```python
from build123d import *

# Parameters (mm, degrees)
F0_R     = 1.5
F1_DEPTH = 2.8448
F2_DEPTH = 1.3208
F3_DEPTH = 0.381
F4_DEPTH = 2.8458


with BuildPart() as f1:
    # F0 (on Top) → F1 (new body)
    with BuildSketch(Plane.XY):
        with BuildLine():
            Line((11.4554, 2.2225), (-11.4554, 2.2225))
            ThreePointArc((-11.4554, 2.2225), (-12.896206, 1.39065), (-12.896206, -0.27305))
            Line((-12.896206, -0.27305), (-12.25096, -1.39065))
            ThreePointArc((-12.25096, -1.39065), (-11.642003, -1.999606), (-10.810153, -2.2225))
            Line((-10.810153, -2.2225), (10.810153, -2.2225))
            ThreePointArc((10.810153, -2.2225), (11.642003, -1.999606), (12.25096, -1.39065))
            Line((12.25096, -1.39065), (12.896206, -0.27305))
            ThreePointArc((12.896206, -0.27305), (12.896206, 1.39065), (11.4554, 2.2225))
        make_face()
        with BuildLine():
            ThreePointArc((-12.566251, -0.08255), (-12.566251, 1.20015), (-11.4554, 1.8415))
            Line((-11.4554, 1.8415), (11.4554, 1.8415))
            ThreePointArc((11.4554, 1.8415), (12.566251, 1.20015), (12.566251, -0.08255))
            Line((12.566251, -0.08255), (11.921004, -1.20015))
            ThreePointArc((11.921004, -1.20015), (11.451503, -1.669651), (10.810153, -1.8415))
            Line((10.810153, -1.8415), (-10.810153, -1.8415))
            ThreePointArc((-10.810153, -1.8415), (-11.451503, -1.669651), (-11.921004, -1.20015))
            Line((-11.921004, -1.20015), (-12.566251, -0.08255))
        make_face(mode=Mode.SUBTRACT)
        with BuildLine():
            Line((11.4554, 1.8415), (-11.4554, 1.8415))
            ThreePointArc((-11.4554, 1.8415), (-12.566251, 1.20015), (-12.566251, -0.08255))
            Line((-12.566251, -0.08255), (-11.921004, -1.20015))
            ThreePointArc((-11.921004, -1.20015), (-11.451503, -1.669651), (-10.810153, -1.8415))
            Line((-10.810153, -1.8415), (10.810153, -1.8415))
            ThreePointArc((10.810153, -1.8415), (11.451503, -1.669651), (11.921004, -1.20015))
            Line((11.921004, -1.20015), (12.566251, -0.08255))
            ThreePointArc((12.566251, -0.08255), (12.566251, 1.20015), (11.4554, 1.8415))
        make_face()
        with BuildLine():
            ThreePointArc((-12.34628, 0.04445), (-12.34628, 1.07315), (-11.4554, 1.5875))
            Line((-11.4554, 1.5875), (11.4554, 1.5875))
            ThreePointArc((11.4554, 1.5875), (12.34628, 1.07315), (12.34628, 0.04445))
            Line((12.34628, 0.04445), (11.701034, -1.07315))
            ThreePointArc((11.701034, -1.07315), (11.324503, -1.44968), (10.810153, -1.5875))
            Line((10.810153, -1.5875), (-10.810153, -1.5875))
            ThreePointArc((-10.810153, -1.5875), (-11.324503, -1.44968), (-11.701034, -1.07315))
            Line((-11.701034, -1.07315), (-12.34628, 0.04445))
        make_face(mode=Mode.SUBTRACT)
        with BuildLine():
            Line((11.4554, 1.5875), (-11.4554, 1.5875))
            ThreePointArc((-11.4554, 1.5875), (-12.34628, 1.07315), (-12.34628, 0.04445))
            Line((-12.34628, 0.04445), (-11.701034, -1.07315))
            ThreePointArc((-11.701034, -1.07315), (-11.324503, -1.44968), (-10.810153, -1.5875))
            Line((-10.810153, -1.5875), (10.810153, -1.5875))
            ThreePointArc((10.810153, -1.5875), (11.324503, -1.44968), (11.701034, -1.07315))
            Line((11.701034, -1.07315), (12.34628, 0.04445))
            ThreePointArc((12.34628, 0.04445), (12.34628, 1.07315), (11.4554, 1.5875))
        make_face()
        with Locations((-10.500578, 0)):
            Circle(F0_R, mode=Mode.SUBTRACT)
        with Locations((10.500578, 0)):
            Circle(F0_R, mode=Mode.SUBTRACT)
        with Locations((-10.500578, 0)):
            Circle(F0_R)
        with Locations((10.500578, 0)):
            Circle(F0_R)
    extrude(amount=-F1_DEPTH)

    # F0 (on Top) → F2 (cut)
    with BuildSketch(Plane.XY):
        with BuildLine():
            Line((11.4554, 1.5875), (-11.4554, 1.5875))
            ThreePointArc((-11.4554, 1.5875), (-12.34628, 1.07315), (-12.34628, 0.04445))
            Line((-12.34628, 0.04445), (-11.701034, -1.07315))
            ThreePointArc((-11.701034, -1.07315), (-11.324503, -1.44968), (-10.810153, -1.5875))
            Line((-10.810153, -1.5875), (10.810153, -1.5875))
            ThreePointArc((10.810153, -1.5875), (11.324503, -1.44968), (11.701034, -1.07315))
            Line((11.701034, -1.07315), (12.34628, 0.04445))
            ThreePointArc((12.34628, 0.04445), (12.34628, 1.07315), (11.4554, 1.5875))
        make_face()
        with Locations((-10.500578, 0)):
            Circle(F0_R, mode=Mode.SUBTRACT)
        with Locations((10.500578, 0)):
            Circle(F0_R, mode=Mode.SUBTRACT)
        with Locations((-10.500578, 0)):
            Circle(F0_R)
        with Locations((10.500578, 0)):
            Circle(F0_R)
    extrude(amount=-F2_DEPTH, mode=Mode.SUBTRACT)

    # F0 (on Top) → F3 (cut)
    with BuildSketch(Plane.XY):
        with BuildLine():
            Line((11.4554, 1.8415), (-11.4554, 1.8415))
            ThreePointArc((-11.4554, 1.8415), (-12.566251, 1.20015), (-12.566251, -0.08255))
            Line((-12.566251, -0.08255), (-11.921004, -1.20015))
            ThreePointArc((-11.921004, -1.20015), (-11.451503, -1.669651), (-10.810153, -1.8415))
            Line((-10.810153, -1.8415), (10.810153, -1.8415))
            ThreePointArc((10.810153, -1.8415), (11.451503, -1.669651), (11.921004, -1.20015))
            Line((11.921004, -1.20015), (12.566251, -0.08255))
            ThreePointArc((12.566251, -0.08255), (12.566251, 1.20015), (11.4554, 1.8415))
        make_face()
        with BuildLine():
            ThreePointArc((-12.34628, 0.04445), (-12.34628, 1.07315), (-11.4554, 1.5875))
            Line((-11.4554, 1.5875), (11.4554, 1.5875))
            ThreePointArc((11.4554, 1.5875), (12.34628, 1.07315), (12.34628, 0.04445))
            Line((12.34628, 0.04445), (11.701034, -1.07315))
            ThreePointArc((11.701034, -1.07315), (11.324503, -1.44968), (10.810153, -1.5875))
            Line((10.810153, -1.5875), (-10.810153, -1.5875))
            ThreePointArc((-10.810153, -1.5875), (-11.324503, -1.44968), (-11.701034, -1.07315))
            Line((-11.701034, -1.07315), (-12.34628, 0.04445))
        make_face(mode=Mode.SUBTRACT)
    extrude(amount=-F3_DEPTH, mode=Mode.SUBTRACT)

    # F0 (on Top) → F4 (cut, through all)
    with BuildSketch(Plane.XY):
        with Locations((-10.500578, 0)):
            Circle(F0_R)
        with Locations((10.500578, 0)):
            Circle(F0_R)
    extrude(amount=-F4_DEPTH, mode=Mode.SUBTRACT)


solid = f1.part
```
Work out the finished part from the listing and answer in its coordinate system (mm). A direction names the side the tool comes from. Round coordinates to 2 decimals unless told otherwise and drop trailing zeros. Write each loop counter-clockwise with the first axis right and the second up, starting at its lowest first coordinate (ties: lowest second). Pieces come first, ordered by that corner, then holes. Notation, with made-up numbers: (-22.5, 7) - (21.5, 7) arc R11 cw to (21.5, 22) - close; hole circle Ø4 at (47, -30.5). An arc over 180 degrees is marked (long way). Return JSON: item names as keys, results as strings. Group by question number.
Q1. Find the intervals of material crossed by L1, parallel to Y at x = 10.5, z = -1.45; L2, parallel to X at y = 1.2, z = -2.35; L3, parallel to Y at x = 8, z = -1, in increasing order.
Q2. The part is cut by section A-A on z = -2.3. Write down the section's boundary in (x, y), then the cut area to 3 significant figures.
Q3. The part is cut by section C-C on y = 1.15. Write down the section's boundary in (x, z).
Q4. The part is cut by section B-B on x = -8.5. Write down the section's boundary in (y, z).
Q5. The part is cut by section D-D on y = -0.55. Write down the section's boundary in (x, z), then the cut area to 3 significant figures.
Q6. Each of these flat-tipped pins is pushed along its axis until it touches: pin 1 Ø1.5 at (x, y) = (-1, 1) entering from +Z; pin 2 Ø2.5 at (x, y) = (-10.5, 0) entering from +Z. Where does it stop, or does it pass through?
Q7. For faces 1 (the flat face through (12.02, -0.52, -0.84)), 2 (the flat face through (12.57, -0.84, -1.4)), determine the directions among +Z, -Z, +X, -X, +Y, -Y from which every point of the face is accessible in a straight line to the end or side of a thin tool.
Q8. The mould has two halves that part along Y. Classify faces 3 (the flat face through (-12.58, -0.82, -1.4)), 4 (the flat face through (0, 2, 0)), 5 (the flat face through (0, -1.588, -1)): released by +Y, released by -Y, zero draft, split by the parting line, or undercut.
Solved:
{
 "1": {"L1": "-2.22 to -1.5, 1.5 to 2.22", "L2": "-12.99 to -11.4, -9.6 to 9.6, 11.4 to 12.99", "L3": "-2.22 to -1.59, 1.59 to 2.22"},
 "2": {"outline": "(-12.9, -0.27) - (-12.25, -1.39) arc R1.66 ccw to (-10.81, -2.22) - (10.81, -2.22) arc R1.66 ccw to (12.25, -1.39) - (12.9, -0.27) arc R1.66 ccw to (11.46, 2.22) - (-11.46, 2.22) arc R1.66 ccw to start; hole circle Ø3 at (-10.5, 0); hole circle Ø3 at (10.5, 0)", "area": "97.8 mm²"},
 "3": {"outline": "(-13.01, -2.84) - (-11.46, -2.84) - (-11.46, -1.32) - (-12.3, -1.32) - (-12.3, -0.38) - (-12.59, -0.38) - (-12.59, 0) - (-13.01, 0) - close; (-9.54, -2.84) - (9.54, -2.84) - (9.54, -1.32) - (-9.54, -1.32) - close; (11.46, -2.84) - (13.01, -2.84) - (13.01, 0) - (12.59, 0) - (12.59, -0.38) - (12.3, -0.38) - (12.3, -1.32) - (11.46, -1.32) - close"},
 "4": {"outline": "(-2.22, -2.84) - (2.22, -2.84) - (2.22, 0) - (1.84, 0) - (1.84, -0.38) - (1.59, -0.38) - (1.59, -1.32) - (-1.59, -1.32) - (-1.59, -0.38) - (-1.84, -0.38) - (-1.84, 0) - (-2.22, 0) - close"},
 "5": {"outline": "(-12.74, -2.84) - (-11.9, -2.84) - (-11.9, -1.32) - (-12, -1.32) - (-12, -0.38) - (-12.3, -0.38) - (-12.3, 0) - (-12.74, 0) - close; (-9.11, -2.84) - (9.11, -2.84) - (9.11, -1.32) - (-9.11, -1.32) - close; (11.9, -2.84) - (12.74, -2.84) - (12.74, 0) - (12.3, 0) - (12.3, -0.38) - (12, -0.38) - (12, -1.32) - (11.9, -1.32) - close", "area": "32.0 mm²"},
 "6": {"pin 1": "z = -0.38", "pin 2": "through"},
 "7": {"face 1": "+Z", "face 2": "+Z, -Z, +X, -Y"},
 "8": {"face 3": "released by -Y", "face 4": "zero draft", "face 5": "undercut"}
}
